Can you work these out from the drawing? Everything is in mm from the part's minimum corner. A direction names the side the tool comes from. Coordinates: 2 decimals unless noted, no trailing zeros. Loops run counter-clockwise (first coordinate to the right, second up) from the corner with the lowest first, then second, coordinate; pieces in that order, holes last. Notation, with made-up numbers: (65.25, 68) - (69.25, 68) arc R21 cw to (69.25, 103) - close; hole circle Ø9 at (-17, 6.5). An arc over 180 degrees is marked (long way). Use CSV: the item, a comma, the result in double quotes.
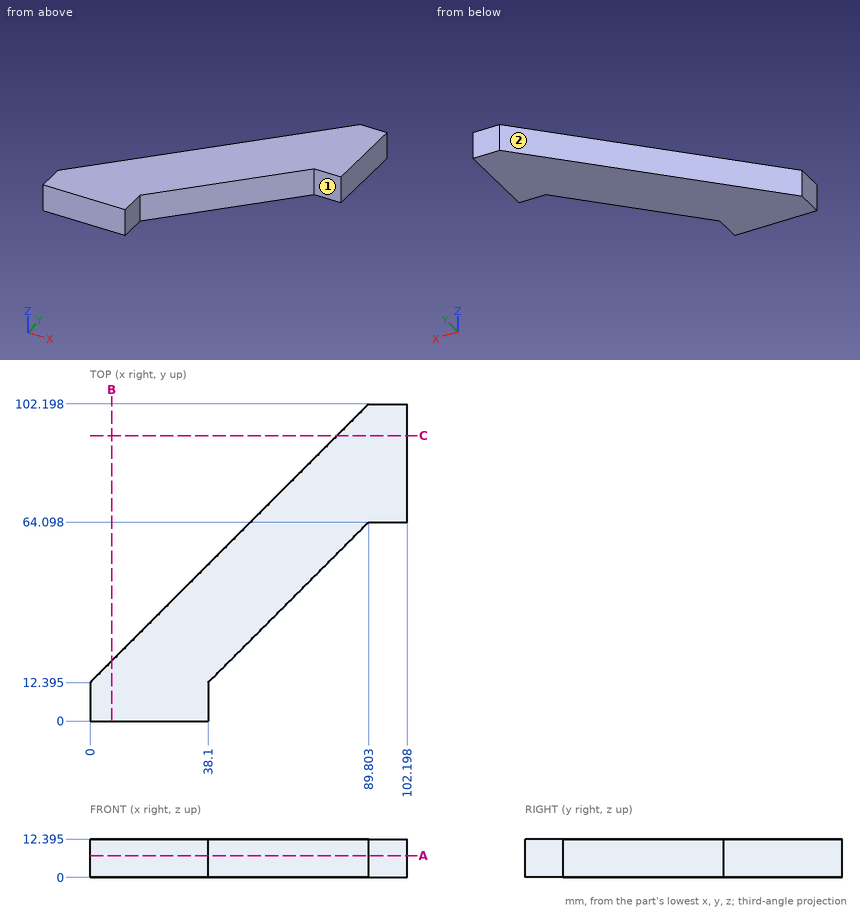
(1) Suppose I cut it at C-C (y = 92). Write out the boundary of the cut face in (x, z) (1 decimal).
Computed:
outline,"(79.6, 0) - (102.2, 0) - (102.2, 12.4) - (79.6, 12.4) - close"
(2) Which directions (+Z, -Z, +X, -X, +Y, -Y) give clear straight access to the entire face, cutting with the end or side of a thin tool? Please do the marked faces 1 and 2.
Computed:
face 1,"+Z, -Z, +X, -Y"
face 2,"+Z, -Z, -X, +Y"
(3) Please list where these lines run through material, in increasing order: line 1 (Y direction, x = 90.5, z = 9.75); line 2 (Y direction, x = 65.5, z = 2) (1 decimal).
Computed:
line 1,"y = 64.1 to 102.2"
line 2,"y = 39.8 to 77.9"
(4) Suppose I cut it at B-B (x = 7). Write out the boundary of the cut face in (y, z) (1 decimal).
Computed:
outline,"(0, 0) - (19.4, 0) - (19.4, 12.4) - (0, 12.4) - close"
(5) Suppose I cut it at A-A (z = 7). Write out the boundary of the cut face in (x, y) (1 decimal).
Computed:
outline,"(0, 0) - (38.1, 0) - (38.1, 12.4) - (89.8, 64.1) - (102.2, 64.1) - (102.2, 102.2) - (89.8, 102.2) - (0, 12.4) - close"
(6) Will these pins go through, and if not, where does the flat tip stop? pin 1 (4 mm diameter, centred on x = 17, y = 17, fed in from -Z); pin 2 (2 mm diameter, centred on y = 70.5, z = 9.5, fed in from -X) (1 decimal); pin 3 (3 mm diameter, centred on y = 15.5, z = 10.5, fed in from +X) (1 decimal).
Computed:
pin 1,"stops at z = 0"
pin 2,"stops at x = 57.1"
pin 3,"stops at x = 42.7"
